The figure shows three views and two pictorial views of one solid part (mm, origin at its lowest corner). Answer the questions. Coordinates: 2 decimals unless noted, no trailing zeros. Loops run counter-clockwise (first coordinate to the right, second up) from the corner with the lowest first, then second, coordinate; pieces in that order, holes last. Notation, with made-up numbers: M 17,-35.75 L 74,-35.75 A22 cw 74,-11.75 Z; hole C -8.5,26.5 d5. An arc over 180 degrees is marked long. Answer as a JSON object with one key per item and string values. Group by question number.
1. Determine the mould class of the marked faces 1, 2, 3 and 4 for opening direction X: released by +X, released by -X, zero draft, split by the parting line, or undercut.
2. Straight lines are drawn through the part: L1, parallel to X at y = 63.5, z = 77.5; L2, parallel to X at y = 94, z = 86.5. For each, find the intervals that lie inside material, in ascending order.
3. A cutting plane is placed at B-B on z = 20. Give the vertices of the cut face in (x, y).
4. Given pin 1 (2 mm diameter, centred on y = 13.5, z = 74.5, fed in from -X); pin 2 (6 mm diameter, centred on x = 98.5, y = 52, fed in from +Z), each flat-ended and moving along its own axis, determine where each tip first touches the part or whether it passes through.
5. A cutting plane is placed at C-C on x = 63.5. Give the vertices of the cut face in (y, z), and give its area (3 significant figures).
6. A cutting plane is placed at A-A on y = 63.5. Give the vertices of the cut face in (x, z).
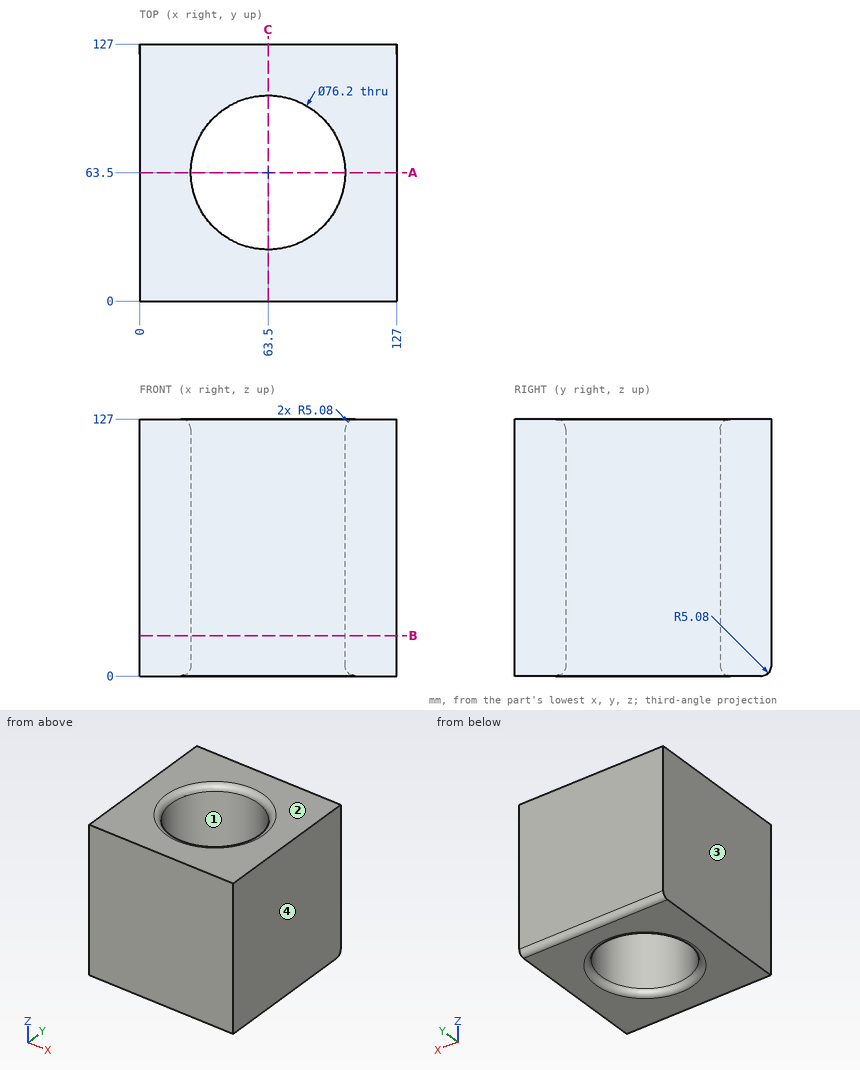
From the geometry:
{
 "1": {"face 1": "undercut", "face 2": "zero draft", "face 3": "released by -X", "face 4": "released by +X"},
 "2": {"L1": "x = 0 to 25.4, 101.6 to 127", "L2": "x = 0 to 40.67, 86.33 to 127"},
 "3": {"outline": "M 0,0 L 127,0 L 127,127 L 0,127 Z; hole C 63.5,63.5 d76.2"},
 "4": {"pin 1": "stops at x = 0", "pin 2": "stops at z = 125.75"},
 "5": {"outline": "M 0,0 L 20.32,0 A5.08 ccw 25.4,5.08 L 25.4,121.92 A5.08 ccw 20.32,127 L 0,127 Z; M 101.6,5.08 A5.08 ccw 106.68,0 L 121.92,0 A5.08 ccw 127,5.08 L 127,127 L 106.68,127 A5.08 ccw 101.6,121.92 Z", "area": "6,420 mm²"},
 "6": {"outline": "M 0,0 L 20.32,0 A5.08 ccw 25.4,5.08 L 25.4,121.92 A5.08 ccw 20.32,127 L 0,127 Z; M 101.6,5.08 A5.08 ccw 106.68,0 L 127,0 L 127,127 L 106.68,127 A5.08 ccw 101.6,121.92 Z"}
}
